Work out the finished part from the listing and answer in its coordinate system (mm). Face numbers are marked on the shaded views. Give positions to 0.01 mm unless a question says otherwise; leave off trailing zeros. Loops run counter-clockwise (first coordinate to the right, second up) from the corner with the lowest first, then second, coordinate; pieces in that order, holes last. Notation, with made-up numbers: M -5,35.25 L 35,35.25 A20 cw 35,43.25 Z; hole C 13,-9 d11. An arc over 180 degrees is marked long. Write item = value, one per line. Start each with the question number.
1. Section D-D on z = -0.8 is taken. Determine the outline of the cut face in (x, y).
2. Section C-C on y = -2 is taken. Determine the outline of the cut face in (x, z) (3 decimals).
3. The mould has two halves that part along X. Classify the marked faces 1, 2 and 3: released by +X, released by -X, zero draft, split by the parting line, or undercut.
4. Consider L1, parallel to X at y = 2.25, z = 0.3; L2, parallel to X at y = -1, z = -0.2 (3 decimals); L3, parallel to X at y = 4.75, z = 0.25. Determine where each line is inside the solid, lowest interval first. Write a range as [from, to].
5. Section B-B on x = 8.25 is taken. Determine the outline of the cut face in (y, z).
6. Section A-A on y = 2.5 is taken. Determine the outline of the cut face in (x, z), plus the area to 3 significant figures.
7. Flat-ended cylindrical pins translate along their axes: pin 1 Ø0.5 at (x, y) = (0, -1.5) entering from +Z (3 decimals); pin 2 Ø0.5 at (y, z) = (-1.5, 0) entering from -X (3 decimals). Find the tip coordinate at first contact, or state that the pin passes through.
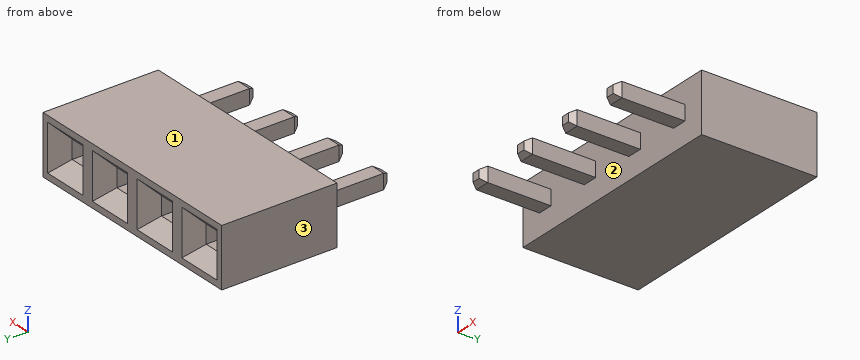
```python
from build123d import *

# Parameters (mm, degrees)
SKETCH1_W                   = 2.54
SKETCH1_H                   = 2.54
BOSS_EXTRUDE1_DEPTH         = 5
SKETCH2_W                   = 0.65
SKETCH2_H                   = 0.65
BOSS_EXTRUDE2_DEPTH         = 3
CHAMFER1_SIZE               = 0.15
CHAMFER1_SIZE2              = 0.259807621
SKETCH3_W                   = 0.8
SKETCH3_H                   = 0.8
CUT_EXTRUDE1_DEPTH          = 3
CHAMFER2_SIZE               = 0.6
LPATTERN1_COUNT             = 4
LPATTERN1_PITCH             = 2.54
CHAMFER1_OF_LPATTERN1_SIZE2 = 0.15
CHAMFER1_OF_LPATTERN1_SIZE  = 0.259807621
CHAMFER2_OF_LPATTERN1_SIZE  = 0.6


with BuildPart() as part:
    # Sketch1 → Boss-Extrude1 (new body)
    with BuildSketch(Plane(origin=(0, 0, 0), x_dir=(1, 0, 0), z_dir=(0, 1, 0))):
        Rectangle(SKETCH1_W, SKETCH1_H)
    boss_extrude1 = extrude(amount=BOSS_EXTRUDE1_DEPTH)

    # Sketch2 → Boss-Extrude2 (add)
    with BuildSketch(Plane.XZ):
        Rectangle(SKETCH2_W, SKETCH2_H)
    boss_extrude2 = extrude(amount=BOSS_EXTRUDE2_DEPTH)

    # Chamfer1
    chamfer1_edges = [part.edges().sort_by_distance(p)[0] for p in [
        (0.325, -3, 0),
        (0, -3, 0.325),
        (-0.325, -3, 0),
        (0, -3, -0.325),
    ]]
    chamfer1_side = [part.faces().sort_by_distance(p)[0] for p in [
        (0, -3, 0),
    ]]
    chamfer(chamfer1_edges, length=CHAMFER1_SIZE, length2=CHAMFER1_SIZE2, reference=chamfer1_side[0])

    # Sketch3 → Cut-Extrude1 (cut)
    with BuildSketch(Plane(origin=(0, 5, 0), x_dir=(1, 0, 0), z_dir=(0, 1, 0))):
        Rectangle(SKETCH3_W, SKETCH3_H)
    cut_extrude1 = extrude(amount=-CUT_EXTRUDE1_DEPTH, mode=Mode.SUBTRACT)

    # Chamfer2
    chamfer2_edges = [part.edges().sort_by_distance(p)[0] for p in [
        (0.4, 5, 0),
        (0, 5, -0.4),
        (-0.4, 5, 0),
        (0, 5, 0.4),
    ]]
    chamfer(chamfer2_edges, length=CHAMFER2_SIZE)

    # LPattern1: Boss-Extrude1, Boss-Extrude2, Cut-Extrude1 ×4
    with Locations(*[(i * LPATTERN1_PITCH, 0, 0) for i in range(1, LPATTERN1_COUNT)]):
        add(boss_extrude1)
        add(boss_extrude2)
        add(cut_extrude1, mode=Mode.SUBTRACT)

    # Chamfer1 of LPattern1
    chamfer1_of_lpattern1_edges = [part.edges().sort_by_distance(p)[0] for p in [
        (2.865, -3, 0),
        (2.54, -3, 0.325),
        (2.215, -3, 0),
        (2.54, -3, -0.325),
        (5.405, -3, 0),
        (5.08, -3, 0.325),
        (4.755, -3, 0),
        (5.08, -3, -0.325),
        (7.945, -3, 0),
        (7.62, -3, 0.325),
        (7.295, -3, 0),
        (7.62, -3, -0.325),
    ]]
    chamfer(chamfer1_of_lpattern1_edges, length=CHAMFER1_OF_LPATTERN1_SIZE, length2=CHAMFER1_OF_LPATTERN1_SIZE2)

    # Chamfer2 of LPattern1
    chamfer2_of_lpattern1_edges = [part.edges().sort_by_distance(p)[0] for p in [
        (2.94, 5, 0),
        (2.54, 5, -0.4),
        (2.14, 5, 0),
        (2.54, 5, 0.4),
        (5.48, 5, 0),
        (5.08, 5, -0.4),
        (4.68, 5, 0),
        (5.08, 5, 0.4),
        (8.02, 5, 0),
        (7.62, 5, -0.4),
        (7.22, 5, 0),
        (7.62, 5, 0.4),
    ]]
    chamfer(chamfer2_of_lpattern1_edges, length=CHAMFER2_OF_LPATTERN1_SIZE)


solid = part.part
```
Verdict:
q1.outline = M -1.27,0 L 8.89,0 L 8.89,5 L 8.62,5 L 8.42,4.8 L 6.82,4.8 L 6.62,5 L 6.08,5 L 5.88,4.8 L 4.28,4.8 L 4.08,5 L 3.54,5 L 3.34,4.8 L 1.74,4.8 L 1.54,5 L 1,5 L 0.8,4.8 L -0.8,4.8 L -1,5 L -1.27,5 Z
q2.outline = M -0.325,-0.325 L 0.325,-0.325 L 0.325,0.325 L -0.325,0.325 Z; M 2.215,-0.325 L 2.865,-0.325 L 2.865,0.325 L 2.215,0.325 Z; M 4.755,-0.325 L 5.405,-0.325 L 5.405,0.325 L 4.755,0.325 Z; M 7.295,-0.325 L 7.945,-0.325 L 7.945,0.325 L 7.295,0.325 Z
q3.face_1 = zero draft
q3.face_2 = undercut
q3.face_3 = released by -X
q4.L1 = [-1.27, -0.4], [0.4, 2.14], [2.94, 4.68], [5.48, 7.22], [8.02, 8.89]
q4.L2 = [-0.325, 0.325], [2.215, 2.865], [4.755, 5.405], [7.295, 7.945]
q4.L3 = [-1.27, -0.75], [0.75, 1.79], [3.29, 4.33], [5.83, 6.87], [8.37, 8.89]
q5.outline = M 0,-1.27 L 5,-1.27 L 5,-1 L 4.63,-0.63 L 4.63,0.63 L 5,1 L 5,1.27 L 0,1.27 Z
q6.outline = M -1.27,-1.27 L 8.89,-1.27 L 8.89,1.27 L -1.27,1.27 Z; hole M -0.4,-0.4 L 0.4,-0.4 L 0.4,0.4 L -0.4,0.4 Z; hole M 2.14,-0.4 L 2.94,-0.4 L 2.94,0.4 L 2.14,0.4 Z; hole M 4.68,-0.4 L 5.48,-0.4 L 5.48,0.4 L 4.68,0.4 Z; hole M 7.22,-0.4 L 8.02,-0.4 L 8.02,0.4 L 7.22,0.4 Z
q6.area = 23.2 mm2
q7.pin_1 = 0.325
q7.pin_2 = -0.325
